Source: CAD feature listing. Evaluate the final solid. Frame: model axes, mm. A direction names the side the tool comes from. Coordinates: 2 decimals unless noted, no trailing zeros. Loops run counter-clockwise (first coordinate to the right, second up) from the corner with the lowest first, then second, coordinate; pieces in that order, holes last. Notation, with made-up numbers: (61.5, 8) - (96.5, 8) arc R21 ccw to (96.5, 12) - close; hole circle Ø5 at (77.25, -29). An arc over 180 degrees is marked (long way). Use CSV: the item, a comma, the result in double quotes. Start each with the question number.
```python
from build123d import *

# Parameters (mm, degrees)
SKETCH_W        = 87
SKETCH_H        = 87
SKETCH_W_2      = 54
SKETCH_H_2      = 54
PAD_DEPTH       = 6
SKETCH001_W     = 84.2
SKETCH001_H     = 84.2
SKETCH001_W_2   = 56.8
SKETCH001_H_2   = 56.8
POCKET_DEPTH    = 4.6
PAD001_DEPTH    = 1.4
SKETCH003_W     = 7.25
SKETCH003_H     = 1.4
PAD002_DEPTH    = 3.3
PAD006_DEPTH    = 1.4
SKETCH004_W     = 30
SKETCH004_H     = 6.5
PAD003_DEPTH    = 1.4
SKETCH005_W     = 30
SKETCH005_H     = 1.4
PAD004_DEPTH    = 11
SKETCH008_R     = 2.5
HOLE001_DEPTH   = 8.001
SKETCH006_W     = 87
SKETCH006_H     = 10
PAD005_DEPTH    = 60
SKETCH007_R     = 2
HOLE_DEPTH      = 54.501
SKETCH009_W     = 84.2
SKETCH009_H     = 57.2
POCKET001_DEPTH = 8
FILLET_R        = 3
FILLET001_R     = 0.5


with BuildPart() as part:
    # Sketch → Pad (new body)
    with BuildSketch(Plane.XY):
        Rectangle(SKETCH_W, SKETCH_H)
        Rectangle(SKETCH_W_2, SKETCH_H_2, mode=Mode.SUBTRACT)
    extrude(amount=PAD_DEPTH)

    # Sketch001 → Pocket (cut)
    with BuildSketch(Plane.XY):
        Rectangle(SKETCH001_W, SKETCH001_H)
        Rectangle(SKETCH001_W_2, SKETCH001_H_2, mode=Mode.SUBTRACT)
    extrude(amount=POCKET_DEPTH, mode=Mode.SUBTRACT)

    # Sketch002 (on DatumPlane) → Pad001 (join)
    with BuildSketch(Plane.XZ.offset(43.5)):
        Polygon((-36.3, 0), (-24.5, 0), (-24.5, -6), (-26.775, -6), (-26.775, -8), (-34.025, -8), (-34.025, -6), (-36.3, -6), align=None)
    pad001 = extrude(amount=-PAD001_DEPTH)

    # Sketch003 (on DatumPlane) → Pad002 (join)
    with BuildSketch(Plane.XZ.offset(43.5)):
        with Locations((-30.4, -7.3)):
            Rectangle(SKETCH003_W, SKETCH003_H)
    pad002 = extrude(amount=PAD002_DEPTH)

    # Sketch010 (on DatumPlane) → Pad006 (join)
    with BuildSketch(Plane.XZ.offset(-43.5)):
        Polygon((-25.5, 0), (-35.2, 0), (-35.2, -6.5), (-32.45, -6.5), (-32.45, -7.85), (-28.25, -7.85), (-28.25, -6.5), (-25.5, -6.5), align=None)
    pad006 = extrude(amount=PAD006_DEPTH)

    # Mirrored002: Pad001, Pad002, Pad006 across Sketch003 V_Axis
    add(pad001.mirror(Plane(origin=(0, -43.5, 0), x_dir=(0, -1, 0), z_dir=(1, 0, 0))))
    add(pad002.mirror(Plane(origin=(0, -43.5, 0), x_dir=(0, -1, 0), z_dir=(1, 0, 0))))
    add(pad006.mirror(Plane(origin=(0, -43.5, 0), x_dir=(0, -1, 0), z_dir=(1, 0, 0))))

    # Sketch004 (on DatumPlane) → Pad003 (join)
    with BuildSketch(Plane.XZ.offset(-43.5)):
        with Locations((0, -3.25)):
            Rectangle(SKETCH004_W, SKETCH004_H)
    extrude(amount=PAD003_DEPTH)

    # Sketch005 (on DatumPlane) → Pad004 (join)
    with BuildSketch(Plane.XZ.offset(-43.5)):
        with Locations((0, -5.8)):
            Rectangle(SKETCH005_W, SKETCH005_H)
    extrude(amount=-PAD004_DEPTH)

    # Sketch008 → Hole001 (cut, through all)
    with BuildSketch(Plane.XY):
        with Locations((0, 49.5)):
            Circle(SKETCH008_R)
    extrude(amount=-HOLE001_DEPTH, mode=Mode.SUBTRACT)

    # Sketch006 (on DatumPlane) → Pad005 (join)
    with BuildSketch(Plane.XY.offset(6)):
        with Locations((0, 38.5)):
            Rectangle(SKETCH006_W, SKETCH006_H)
    extrude(amount=PAD005_DEPTH)

    # Sketch007 → Hole (cut, through all)
    with BuildSketch(Plane.XZ):
        with Locations((-32.5, 52)):
            Circle(SKETCH007_R)
        with Locations((32.5, 52)):
            Circle(SKETCH007_R)
        with Locations((-32.5, 18)):
            Circle(SKETCH007_R)
        with Locations((32.5, 18)):
            Circle(SKETCH007_R)
    extrude(amount=-HOLE_DEPTH, mode=Mode.SUBTRACT)

    # Sketch009 (on DatumPlane) → Pocket001 (cut)
    with BuildSketch(Plane.XZ.offset(-43.5)):
        with Locations((0, 36)):
            Rectangle(SKETCH009_W, SKETCH009_H)
    extrude(amount=POCKET001_DEPTH, mode=Mode.SUBTRACT)

    # Fillet
    fillet_edges = [part.edges().sort_by_distance(p)[0] for p in [
        (43.5, 38.5, 66),
        (-43.5, 38.5, 66),
        (-42.1, 39.5, 64.6),
        (42.1, 39.5, 64.6),
        (42.1, 39.5, 7.4),
        (-42.1, 39.5, 7.4),
        (0, 33.5, 6),
    ]]
    fillet(fillet_edges, radius=FILLET_R)

    # Fillet001
    fillet001_edges = [part.edges().sort_by_distance(p)[0] for p in [
        (0, 43.5, -5.1),
        (0, 42.1, -6.5),
        (30.4, -43.5, -6.6),
        (-30.4, -43.5, -6.6),
        (-30.4, -42.1, -8),
        (30.4, -42.1, -8),
    ]]
    fillet(fillet001_edges, radius=FILLET001_R)


solid = part.part
```
(1) Pin query (flat end, axial travel): pin 1 Ø1.1 at (x, y) = (25.5, -42.5) entering from -Z; pin 2 Ø0.7 at (x, y) = (31, 43) entering from -Z; pin 3 Ø1.1 at (x, y) = (-33.5, 43) entering from -Z. Return the tip coordinate at first contact, or that it passes through.
(2) Section A-A on x = 7. Output: boundary loops of the cut face in (y, z).
(3) Draft query along Y for faces 1 (the cylindrical face through (0.61, 32.64, 6.9)), 2 (the flat face through (-27, 0, 3)), 3 (the flat face through (-1, 40, 64.6)). Return one class per face: released by +Y, released by -Y, zero draft, split by the parting line, or undercut.
(4) Section D-D on y = 40. Output: boundary loops of the cut face in (x, z).
(5) Ray query, line 1 (Z direction, x = -32.5, y = 35.05); line 2 (Y direction, x = -10.5, z = 4); line 3 (Z direction, x = -1, y = 38.5). Return the intervals inside material, ascending. Write a range as [from, to].
(6) Section C-C on z = 52. Output: boundary loops of the cut face in (x, y), plus the area to 3 significant figures.
(7) Reachability of faces 4 (the flat face through (-42.1, 40, 36)), 5 (the flat face through (-1, -42.1, 1)), 6 (the flat face through (27, 0, 3)), 7 (the flat face through (30, -45, -6.6)), 8 (the flat face through (-2.2, -27.2, 0)) from +Z, -Z, +X, -X, +Y, -Y: full face, straight path, thin tool, end or side. Return the list, or none.
(8) Section B-B on y = -13. Output: boundary loops of the cut face in (x, z).
Solution:
1,pin 1,"stops at z = -6"
1,pin 2,"stops at z = -7.85"
1,pin 3,"stops at z = -6.5"
2,outline,"(-43.5, 0) - (-42.1, 0) - (-42.1, 4.6) - (-28.4, 4.6) - (-28.4, 0) - (-27, 0) - (-27, 6) - (-43.5, 6) - close; (27, 0) - (28.4, 0) - (28.4, 4.6) - (42.1, 4.6) - (42.1, -6) arc R0.5 ccw to (42.6, -6.5) - (54.5, -6.5) - (54.5, -5.1) - (44, -5.1) arc R0.5 cw to (43.5, -4.6) - (43.5, 7.4) - (35.5, 7.4) - (35.5, 64.6) - (43.5, 64.6) - (43.5, 66) - (33.5, 66) - (33.5, 9) arc R3 cw to (30.5, 6) - (27, 6) - close"
3,face 1,"released by -Y"
3,face 2,"undercut"
3,face 3,"zero draft"
4,outline,"(-43.5, 0) - (-42.1, 0) - (-42.1, 4.6) - (42.1, 4.6) - (42.1, 0) - (43.5, 0) - (43.5, 63) arc R3 ccw to (40.5, 66) - (-40.5, 66) arc R3 ccw to (-43.5, 63) - close; hole (-42.1, 10.4) arc R3 ccw to (-39.1, 7.4) - (39.1, 7.4) arc R3 ccw to (42.1, 10.4) - (42.1, 61.6) arc R3 ccw to (39.1, 64.6) - (-39.1, 64.6) arc R3 ccw to (-42.1, 61.6) - close"
5,line 1,"z = [4.6, 16], [20, 50], [54, 66]"
5,line 2,"y = [-43.5, -42.1], [-28.4, -27], [27, 28.4], [42.1, 43.5]"
5,line 3,"z = [4.6, 7.4], [64.6, 66]"
6,outline,"(-43.5, 33.5) - (-34.5, 33.5) - (-34.5, 35.5) - (-42.1, 35.5) - (-42.1, 43.5) - (-43.5, 43.5) - close; (-30.5, 33.5) - (30.5, 33.5) - (30.5, 35.5) - (-30.5, 35.5) - close; (34.5, 33.5) - (43.5, 33.5) - (43.5, 43.5) - (42.1, 43.5) - (42.1, 35.5) - (34.5, 35.5) - close"
6,area,"180 mm²"
7,face 4,"+Y"
7,face 5,"-Z"
7,face 6,"+Z, -Z"
7,face 7,"+Z, +X, -X, -Y"
7,face 8,"-Z, +X, -X"
8,outline,"(-43.5, 0) - (-42.1, 0) - (-42.1, 4.6) - (-28.4, 4.6) - (-28.4, 0) - (-27, 0) - (-27, 6) - (-43.5, 6) - close; (27, 0) - (28.4, 0) - (28.4, 4.6) - (42.1, 4.6) - (42.1, 0) - (43.5, 0) - (43.5, 6) - (27, 6) - close"
